Work out the finished part from the listing and answer in its coordinate system (mm). Face numbers are marked on the shaded views. A direction names the side the tool comes from. Round coordinates to 2 decimals unless told otherwise and drop trailing zeros. Loops run counter-clockwise (first coordinate to the right, second up) from the corner with the lowest first, then second, coordinate; pieces in that order, holes last. Notation, with made-up numbers: M -19,-39 L 7,-39 A22 cw 7,-25 Z; hole C 1.25,-13 d9. An arc over 180 degrees is marked long. One line per item, written item: value.
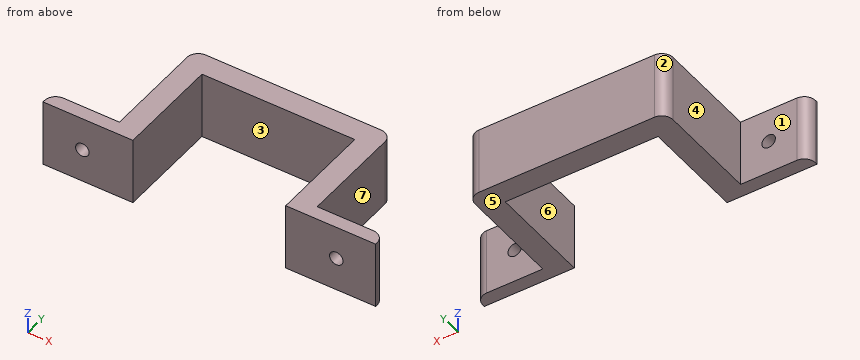
```python
from build123d import *

# Parameters (mm, degrees)
BOSS_EXTRUDE1_DEPTH = 15
FILLET1_R           = 2.5
SKETCH2_R           = 1.5
CUT_EXTRUDE1_DEPTH  = 3


with BuildPart() as part:
    # Sketch1 → Boss-Extrude1 (new body)
    with BuildSketch(Plane.XY):
        Polygon((17, 23), (-17, 23), (-17, 0), (-37, 0), (-37, 3), (-22, 3), (-22, 28), (22, 28), (22, 3), (37, 3), (37, 0), (17, 0), align=None)
    extrude(amount=BOSS_EXTRUDE1_DEPTH)

    # Fillet1
    fillet1_edges = [part.edges().sort_by_distance(p)[0] for p in [
        (-37, 3, 7.5),
        (-22, 28, 7.5),
        (22, 28, 7.5),
        (37, 3, 7.5),
    ]]
    fillet(fillet1_edges, radius=FILLET1_R)

    # Sketch2 → Cut-Extrude1 (cut)
    with BuildSketch(Plane(origin=(0, 3, 0), x_dir=(1, 0, 0), z_dir=(0, 1, 0))):
        with Locations(Location((-28.25, -7.5, 0), (0, 0, 270))):
            Circle(SKETCH2_R)
        with Locations(Location((28.25, -7.5, 0), (0, 0, 270))):
            Circle(SKETCH2_R)
    extrude(amount=-CUT_EXTRUDE1_DEPTH, mode=Mode.SUBTRACT)


solid = part.part
```
1) The mould has two halves that part along X. Classify the marked faces 1, 2 and 3: +X half, -X half, draft (parallel to the pull), parting line (faces both ways), or undercut.
Check values:
face 1: draft
face 2: -X half
face 3: undercut
2) Find the intervals of material crossed by probe 1 along X at (y, z) = (0.65, 7.5); probe 2 along X at (y, z) = (14.5, 5); probe 3 along X at (y, z) = (1.45, 7.5), in increasing order. Write a range as from..to.
Check values:
probe 1: -37..-29.75, -26.75..-17, 17..26.75, 29.75..37
probe 2: -22..-17, 17..22
probe 3: -36.81..-29.75, -26.75..-17, 17..26.75, 29.75..36.81
3) Find section D-D (z = 2.25). Give the vertices of the cut face in (x, y).
Check values:
outline: M -37,0 L -17,0 L -17,23 L 17,23 L 17,0 L 37,0 L 37,0.5 A2.5 ccw 34.5,3 L 22,3 L 22,25.5 A2.5 ccw 19.5,28 L -19.5,28 A2.5 ccw -22,25.5 L -22,3 L -34.5,3 A2.5 ccw -37,0.5 Z
4) Find section A-A (x = -28.25). Give the vertices of the cut face in (y, z), then the cut area to 3 significant figures.
Check values:
outline: M 0,0 L 3,0 L 3,6 L 0,6 Z; M 0,9 L 3,9 L 3,15 L 0,15 Z
area: 36.0 mm2
5) For the marked faces 4, 5, 6 and 7, determine the directions among +Z, -Z, +X, -X, +Y, -Y from which every point of the face is accessible in a straight line to the end or side of a thin tool.
Check values:
face 4: +Z, -Z, -X, +Y
face 5: -Z, +X, -X, +Y, -Y
face 6: +Z, -Z, -Y
face 7: +Z, -Z, +X, +Y
6) Find section B-B (y = 14). Give the vertices of the cut face in (x, z), then the cut area to 3 significant figures.
Check values:
outline: M -22,0 L -17,0 L -17,15 L -22,15 Z; M 17,0 L 22,0 L 22,15 L 17,15 Z
area: 150 mm2
7) Each of these flat-tipped pins is pushed along its axis until it touches: pin 1 (2 mm diameter, centred on x = 24, y = 19, fed in from -Z) (1 decimal); pin 2 (7.5 mm diameter, centred on x = -4, z = 7, fed in from -Y); pin 3 (3 mm diameter, centred on y = 20, z = 7.5, fed in from -X); pin 4 (8 mm diameter, centred on y = 9.5, z = 9.5, fed in from +X). Where does it stop, or does it pass through?
Check values:
pin 1: through
pin 2: y = 23
pin 3: x = -22
pin 4: x = 22
8) Find section C-C (z = 7.5). Give the vertices of the cut face in (x, y).
Check values:
outline: M -37,0 L -29.75,0 L -29.75,3 L -34.5,3 A2.5 ccw -37,0.5 Z; M -26.75,0 L -17,0 L -17,23 L 17,23 L 17,0 L 26.75,0 L 26.75,3 L 22,3 L 22,25.5 A2.5 ccw 19.5,28 L -19.5,28 A2.5 ccw -22,25.5 L -22,3 L -26.75,3 Z; M 29.75,0 L 37,0 L 37,0.5 A2.5 ccw 34.5,3 L 29.75,3 Z
